Design review of the part built by this model. Coordinates are the model's own, in mm. A direction names the side the tool comes from. Coordinates: 2 decimals unless noted, no trailing zeros. Order: outer loops, then holes, each group sorted by start corner. A loop starts at its lowest first (then second) coordinate and runs counter-clockwise, first axis right, second up. Notation, with made-up numbers: (-37.5, -27.75) -> (0.5, -27.75) arc R11 cw to (0.5, -19.75) -> close; hole circle Ø3 at (23.5, 41). An arc over 180 degrees is marked (long way). Use a Markdown table: item, result. Add a question column.
Q1. Insertion check: pin 1 (4 mm diameter, centred on x = 255.5, z = 18.5, fed in from -Y); pin 2 (1.5 mm diameter, centred on x = 166, z = 13.5, fed in from +Y). Each pin has a flat end and moves straight along its axis. Give the tip position at first contact, or say it passes through.
Q2. The part is to be moulded in two halves that separate along Z. For faces 6 (the face through (246, -26.479, 16)), 7 (the face through (0, -26, 16)), 8 (the face through (246, -29, 10.108)), say which applies: pulls with the +Z half, pulls with the -Z half, needs draft (parallel to the pull), parting line crosses it, or undercut.
Q3. Machinability: for faces 1 (the face through (246, -28, 22.053)), 2 (the face through (246, -30.479, 16)), 3 (the face through (246, -31.479, 16)), 4 (the face through (246, -25.479, 16)), 5 (the face through (500, -26, 16)), which of the approach directions +Z, -Z, +X, -X, +Y, -Y give a long, thin tool a straight path to every point of the face, cutting with its end or side? Answer none if there is none.
Q4. Add section C-C (x = 335). State the section outline as (y, z) points, then the cut area to 3 significant figures.
Q5. Add section B-B (z = 15.25). State the section outline as (x, y) points, then the cut area to 3 significant figures.
Q6. Add section A-A (y = -28). State the section outline as (x, z) points.
Q7. Wall thickness on probe 1 along Y at (x, z) = (316, 14.75); probe 2 along Z at (x, y) = (147, -33): over which ranges is each line inside the solid? List them lowest first.
from build123d import *

# Parameters (mm, degrees)
F0_W     = 4
F0_H     = 9.9456192771
F1_DEPTH = 500


with BuildPart() as f1:
    # F0 (on Right) → F1 (new body)
    with BuildSketch(Plane.YZ):
        Polygon((-23.479051888, 22.0532231033), (-33.479051888, 22.0532231033), (-33.479051888, 21.0532231033), (-31.479051888, 21.0532231033), (-31.479051888, 11.1076038262), (-33.479051888, 11.1076038262), (-33.479051888, 10.1076038262), (-23.479051888, 10.1076038262), (-23.479051888, 11.1076038262), (-25.479051888, 11.1076038262), (-25.479051888, 21.0532231033), (-23.479051888, 21.0532231033), align=None)
        with Locations((-28.479051888, 16.0804134647)):
            Rectangle(F0_W, F0_H, mode=Mode.SUBTRACT)
    extrude(amount=F1_DEPTH)


solid = f1.part
Established:
| question | item | result |
|---|---|---|
| 1 | pin 1 | y = -31.48 |
| 1 | pin 2 | y = -25.48 |
| 2 | face 6 | undercut |
| 2 | face 7 | needs draft |
| 2 | face 8 | pulls with the -Z half |
| 3 | face 1 | +Z, +X, -X, +Y, -Y |
| 3 | face 2 | +X, -X |
| 3 | face 3 | +X, -X, -Y |
| 3 | face 4 | +X, -X, +Y |
| 3 | face 5 | +Z, -Z, +X, +Y, -Y |
| 4 | outline | (-33.48, 10.11) -> (-23.48, 10.11) -> (-23.48, 11.11) -> (-25.48, 11.11) -> (-25.48, 21.05) -> (-23.48, 21.05) -> (-23.48, 22.05) -> (-33.48, 22.05) -> (-33.48, 21.05) -> (-31.48, 21.05) -> (-31.48, 11.11) -> (-33.48, 11.11) -> close; hole (-30.48, 11.11) -> (-26.48, 11.11) -> (-26.48, 21.05) -> (-30.48, 21.05) -> close |
| 4 | area | 39.9 mm^2 |
| 5 | outline | (0, -31.48) -> (500, -31.48) -> (500, -30.48) -> (0, -30.48) -> close; (0, -26.48) -> (500, -26.48) -> (500, -25.48) -> (0, -25.48) -> close |
| 5 | area | 1,000 mm^2 |
| 6 | outline | (0, 10.11) -> (500, 10.11) -> (500, 11.11) -> (0, 11.11) -> close; (0, 21.05) -> (500, 21.05) -> (500, 22.05) -> (0, 22.05) -> close |
| 7 | probe 1 | -31.48 to -30.48, -26.48 to -25.48 |
| 7 | probe 2 | 10.11 to 11.11, 21.05 to 22.05 |
